Autodesk Fusion 360 part; units mm, degrees
sketch "Schizzo1" plane through (0, 0, 0) normal (0, 0, 1) x (1, 0, 0)
  line L0 (39.554, 71.8617) -> (66.804, 71.8617)
  line L1 (66.804, 71.8617) -> (66.804, 61.8617)
  line L2 (66.804, 61.8617) -> (39.554, 61.8617)
  line L3 (39.554, 61.8617) -> (39.554, 71.8617)
  line L4 (8.0104, 18.4694) -> (37.0104, 18.4694) construction
  line L5 (37.0104, 18.4694) -> (37.0104, 6.4694) construction
  line L6 (37.0104, 6.4694) -> (8.0104, 6.4694) construction
  line L7 (8.0104, 6.4694) -> (8.0104, 18.4694) construction
  line L8 (22.5104, 18.4694) -> (22.5104, 6.4694) construction
  line L9 (8.0104, 12.4694) -> (37.0104, 12.4694) construction
  circle A0 centre (14.5104, 12.4694) radius 1.9
  circle A1 centre (30.5104, 12.4694) radius 1.9
  line L10 (36.9104, 6.5694) -> (8.1104, 6.5694)
  line L11 (8.1104, 6.5694) -> (8.1104, 18.3694)
  line L12 (8.1104, 18.3694) -> (36.9104, 18.3694)
  line L13 (36.9104, 18.3694) -> (36.9104, 6.5694)
  line L14 (36.9104, 6.5694) -> (8.1104, 18.3694) construction
  line L15 (8.1104, 6.5694) -> (36.9104, 18.3694) construction
  point P0 (22.5104, 12.4694)
  dimension "d1" = 27.25
  dimension "d2" = 10
  dimension "d3" = 29
  dimension "d4" = 12
  dimension "d5" = 3.8
  dimension "d6" = 16
  dimension "d7" = 0.1
  dimension "d8" = 0.1
extrude "Estrusione1" add sketch "Schizzo1" along normal blind 0.8 contours L10 L11 L12 L13
extrude "Estrusione2" add sketch "Schizzo1" along normal blind 4 contours A0 | A1
equation "d5 = 4 mm - 0.2 mm"
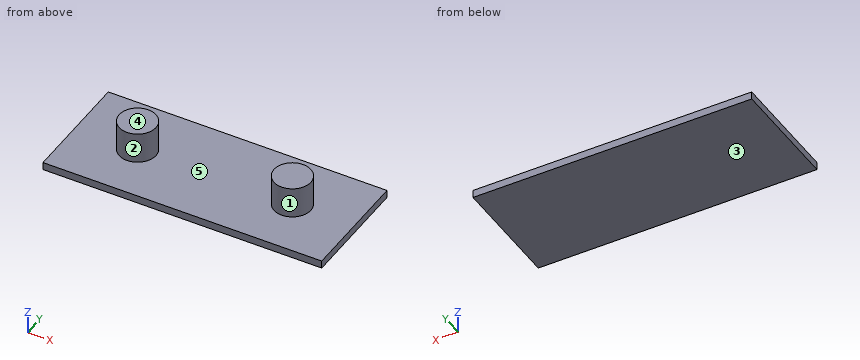
Design review of the part built by this model. Coordinates are the model's own, in mm. Face numbers are marked on the shaded views. A direction names the side the tool comes from. Give positions to 0.01 mm unless a question says otherwise; leave off trailing zeros. Write each loop counter-clockwise with the first axis right and the second up, starting at its lowest first coordinate (ties: lowest second). Pieces come first, ordered by that corner, then holes. Notation, with made-up numbers: (5, -39) - (37, -39) arc R31 ccw to (37, -2) - close; hole circle Ø9 at (89, 22). An arc over 180 degrees is marked (long way). Return JSON: item names as keys, results as strings. Group by question number.
(1) To check wall thickness, follow probe 1 along Z at (x, y) = (27.5, 10.25); probe 2 along X at (y, z) = (11.5, 3.2); probe 3 along X at (y, z) = (12.75, 3.7). State the ranges of each line that lie inside material, in increasing order.
(2) We need section B-B, the plane y = 16.5. Give the boundary of the cut face in (x, z), then the cut area to 3 significant figures.
(3) Mouldability with a two-part tool opening along X and no side actions: class the marked faces 1, 2 and 3 as +X half, -X half, draft (parallel to the pull), parting line (faces both ways), or undercut.
(4) Machinability: for the marked faces 4 and 5, which of the approach directions +Z, -Z, +X, -X, +Y, -Y give a long, thin tool a straight path to every point of the face, cutting with its end or side? Answer none if there is none.
(5) We need section D-D, the plane x = 30. Give the boundary of the cut face in (y, z), then the cut area to 3 significant figures.
(6) We need section A-A, the plane x = 16. Give the boundary of the cut face in (y, z).
(7) We need section C-C, the plane z = 1.6. Give the boundary of the cut face in (x, y), then the cut area to 3 significant figures.
(8) Insertion check: pin 1 (1.5 mm diameter, centred on y = 13.5, z = 2, fed in from -X); pin 2 (2 mm diameter, centred on y = 10.5, z = 2.5, fed in from +X). Each pin has a flat end and moves straight along its axis. Give the tip position at first contact, or say it passes through.
Reported:
{
 "1": {"probe 1": "z = 0 to 0.8", "probe 2": "x = 12.88 to 16.14, 28.88 to 32.14", "probe 3": "x = 12.63 to 16.39, 28.63 to 32.39"},
 "2": {"outline": "(8.11, 0) - (36.91, 0) - (36.91, 0.8) - (8.11, 0.8) - close", "area": "23.0 mm2"},
 "3": {"face 1": "undercut", "face 2": "undercut", "face 3": "draft"},
 "4": {"face 4": "+Z, +X, -X, +Y, -Y", "face 5": "+Z"},
 "5": {"outline": "(6.57, 0) - (18.37, 0) - (18.37, 0.8) - (14.3, 0.8) - (14.3, 4) - (10.64, 4) - (10.64, 0.8) - (6.57, 0.8) - close", "area": "21.2 mm2"},
 "6": {"outline": "(6.57, 0) - (18.37, 0) - (18.37, 0.8) - (13.65, 0.8) - (13.65, 4) - (11.29, 4) - (11.29, 0.8) - (6.57, 0.8) - close"},
 "7": {"outline": "circle Ø3.8 at (14.51, 12.47); circle Ø3.8 at (30.51, 12.47)", "area": "22.7 mm2"},
 "8": {"pin 1": "stops at x = 12.63", "pin 2": "stops at x = 32.14"}
}
